Check sheet for the modelled part. Datum: model origin and axes. Units: mm. Face numbers are marked on the shaded views. Coordinates: 2 decimals unless noted, no trailing zeros. Order: outer loops, then holes, each group sorted by start corner. A loop starts at its lowest first (then second) coordinate and runs counter-clockwise, first axis right, second up.
1. Cross-section at A-A (y = 0). Enter the section's corners in (x, z), then the cut area to 3 significant figures.
2. Cross-section at C-C (x = 19.5). Enter the section's corners in (y, z), then the cut area to 3 significant figures.
3. Thickness scan on line 1 (Y direction, x = 23.2, z = 0); line 2 (X direction, y = -0.75, z = 1.5); line 3 (Z direction, x = 17, y = 2.5). Record the ranges inside material, lowest first.
4. Draft check along Y on the marked faces 1, 2 and 3. Enter one of: released by +Y, released by -Y, zero draft, split by the parting line, or undercut.
5. Gauge pin test, flat ends, axial feed: pin 1 Ø1.5 at (y, z) = (2, -1.5) entering from +X; pin 2 Ø1 at (x, y) = (17.5, 2.5) entering from +Z; pin 3 Ø1 at (y, z) = (-2, -2.5) entering from -X; pin 4 Ø4 at (x, y) = (3.5, 2.5) entering from +Z. Record the tip position at first contact, or that the pin passes through.
```python
from build123d import *

# Parameters (mm, degrees)
SKETCH1_R      = 4.5
EXTRUDE1_DEPTH = 24
FILLET1_R      = 0.5
SKETCH2_R      = 3
EXTRUDE2_DEPTH = 1
FILLET2_R      = 0.5


with BuildPart() as part:
    # Sketch1 → Extrude1 (new body)
    with BuildSketch(Plane(origin=(0, 0, 0), x_dir=(0, 0, -1), z_dir=(1, 0, 0))):
        Circle(SKETCH1_R)
    extrude(amount=EXTRUDE1_DEPTH)

    # Fillet1
    fillet1_edges = [part.edges().sort_by_distance(p)[0] for p in [
        (0, 0, 4.5),
    ]]
    fillet(fillet1_edges, radius=FILLET1_R)

    # Sketch2 → Extrude2 (cut)
    with BuildSketch(Plane(origin=(24, 0, 0), x_dir=(0, 0, -1), z_dir=(1, 0, 0))):
        Circle(SKETCH2_R)
    extrude(amount=-EXTRUDE2_DEPTH, mode=Mode.SUBTRACT)

    # Fillet2
    fillet2_edges = [part.edges().sort_by_distance(p)[0] for p in [
        (24, 0, 4.5),
        (24, 0, 3),
    ]]
    fillet(fillet2_edges, radius=FILLET2_R)


solid = part.part
```
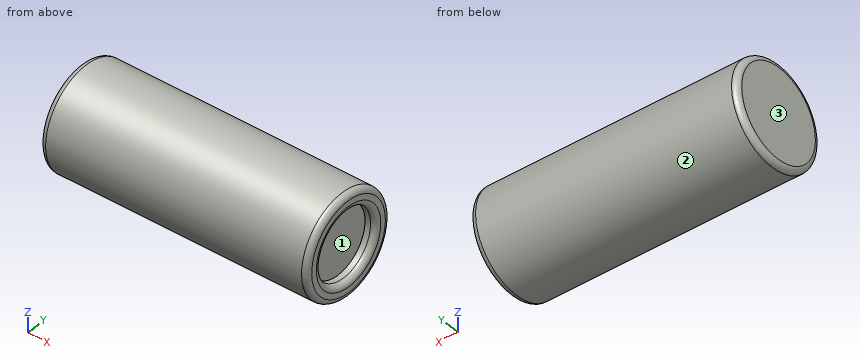
Data:
1. outline: (0, -4) arc R0.5 ccw to (0.5, -4.5) - (23.5, -4.5) arc R0.5 ccw to (24, -4) - (24, -3.5) arc R0.5 ccw to (23.5, -3) - (23, -3) - (23, 3) - (23.5, 3) arc R0.5 ccw to (24, 3.5) - (24, 4) arc R0.5 ccw to (23.5, 4.5) - (0.5, 4.5) arc R0.5 ccw to (0, 4) - close
1. area: 210 mm2
2. outline: circle Ø9 at (0, 0)
2. area: 63.6 mm2
3. line 1: y = -4.5 to -3, 3 to 4.5
3. line 2: x = 0 to 23
3. line 3: z = -3.74 to 3.74
4. face 1: undercut
4. face 2: split by the parting line
4. face 3: zero draft
5. pin 1: stops at x = 23.93
5. pin 2: stops at z = 4.03
5. pin 3: stops at x = 0
5. pin 4: stops at z = 4.47
